Verification items for the finished model (mm, model axes). A direction names the side the tool comes from. Round coordinates to 2 decimals unless told otherwise and drop trailing zeros. Loops run counter-clockwise (first coordinate to the right, second up) from the corner with the lowest first, then second, coordinate; pieces in that order, holes last. Notation, with made-up numbers: M 12,-16.5 L 69,-16.5 A24 cw 69,5.5 Z; hole C -24.75,-6 d10. An arc over 180 degrees is marked long. Answer as CSV lines item,"result".
```python
from build123d import *

# Parameters (mm, degrees)
SKETCH1_W                = 6
SKETCH1_H                = 6
BOSS_EXTRUDE1_DEPTH      = 14
SKETCH2_W                = 1
SKETCH2_H                = 6
SKETCH2_W_2              = 1.5
BOSS_EXTRUDE2_DEPTH      = 10
FILLET1_R                = 3
SKETCH3_R                = 1.5
CUT_EXTRUDE1_DEPTH       = 10
CHAMFER1_SIZE            = 1
CHAMFER2_SIZE            = 1
FILLET1_OF_MIRROR2_R     = 3
CHAMFER1_OF_MIRROR2_SIZE = 1
SKETCH4_R                = 1.25
CUT_EXTRUDE2_DEPTH       = 13
CHAMFER3_SIZE            = 1
CUT_EXTRUDE3_DEPTH       = 10
CUT_EXTRUDE3_DEPTH_BACK  = 10
SKETCH5_W                = 10
SKETCH5_H                = 0.25
CUT_EXTRUDE4_DEPTH       = 10
CUT_EXTRUDE4_DEPTH_BACK  = 10
SKETCH6_W                = 10
SKETCH6_H                = 0.25
CHAMFER4_SIZE            = 1


with BuildPart() as part:
    # Sketch1 → Boss-Extrude1 (new body)
    with BuildSketch(Plane(origin=(0, 0, 0), x_dir=(0, 0, -1), z_dir=(1, 0, 0))):
        Rectangle(SKETCH1_W, SKETCH1_H)
    boss_extrude1 = extrude(amount=BOSS_EXTRUDE1_DEPTH)

    # Sketch2 → Boss-Extrude2 (add)
    with BuildSketch(Plane(origin=(14, 0, 0), x_dir=(0, 0, -1), z_dir=(1, 0, 0))):
        with Locations((3.5, 0)):
            Rectangle(SKETCH2_W, SKETCH2_H)
        with Locations((2.25, 0)):
            Rectangle(SKETCH2_W_2, SKETCH2_H)
    boss_extrude2 = extrude(amount=BOSS_EXTRUDE2_DEPTH)

    # Fillet1
    fillet1_edges = [part.edges().sort_by_distance(p)[0] for p in [
        (24, 3, -2.75),
        (24, -3, -2.75),
    ]]
    fillet(fillet1_edges, radius=FILLET1_R - 0.0001)  # a hair under: the kernel refuses the full size

    # Sketch3 → Cut-Extrude1 (cut)
    with BuildSketch(Plane(origin=(0, 0, -4), x_dir=(-1, 0, 0), z_dir=(0, 0, -1))):
        with Locations((-21, 0)):
            Circle(SKETCH3_R)
    cut_extrude1 = extrude(amount=-CUT_EXTRUDE1_DEPTH, mode=Mode.SUBTRACT)

    # Chamfer1
    chamfer1_edges = [part.edges().sort_by_distance(p)[0] for p in [
        (14, 0, -4),
    ]]
    chamfer(chamfer1_edges, length=CHAMFER1_SIZE - 0.0001)  # a hair under: the kernel refuses the full size

    # Chamfer2
    chamfer2_edges = [part.edges().sort_by_distance(p)[0] for p in [
        (14, 3, 0.75),
        (14, -3, 0.75),
    ]]
    chamfer(chamfer2_edges, length=CHAMFER2_SIZE)

    # Mirror2: Boss-Extrude1, Boss-Extrude2, Cut-Extrude1 across plane
    add(boss_extrude1.mirror(Plane(origin=(0, 0, 0), x_dir=(1, 0, 0), z_dir=(0, 0, -1))))
    add(boss_extrude2.mirror(Plane(origin=(0, 0, 0), x_dir=(1, 0, 0), z_dir=(0, 0, -1))))
    add(cut_extrude1.mirror(Plane(origin=(0, 0, 0), x_dir=(1, 0, 0), z_dir=(0, 0, -1))), mode=Mode.SUBTRACT)

    # Fillet1 of Mirror2
    fillet1_of_mirror2_edges = [part.edges().sort_by_distance(p)[0] for p in [
        (24, 3, 2.75),
        (24, -3, 2.75),
    ]]
    fillet(fillet1_of_mirror2_edges, radius=FILLET1_OF_MIRROR2_R - 0.0001)  # a hair under: the kernel refuses the full size

    # Chamfer1 of Mirror2
    chamfer1_of_mirror2_edges = [part.edges().sort_by_distance(p)[0] for p in [
        (14, 0, 4),
    ]]
    chamfer(chamfer1_of_mirror2_edges, length=CHAMFER1_OF_MIRROR2_SIZE - 0.0001)  # a hair under: the kernel refuses the full size

    # Sketch4 → Cut-Extrude2 (cut)
    with BuildSketch(Plane.ZY):
        Circle(SKETCH4_R)
    extrude(amount=-CUT_EXTRUDE2_DEPTH, mode=Mode.SUBTRACT)

    # Chamfer3
    chamfer3_edges = [part.edges().sort_by_distance(p)[0] for p in [
        (14, -3, 0),
        (14, 3, 0),
    ]]
    chamfer(chamfer3_edges, length=CHAMFER3_SIZE)

    # Sketch5 → Cut-Extrude3 (cut, two sides: drawn at the far end of the back side and taken through both)
    with BuildSketch(Plane(origin=(0, 0, 0), x_dir=(1, 0, 0), z_dir=(0, 1, 0)).offset(-CUT_EXTRUDE3_DEPTH_BACK)):
        with Locations((19, -1.625)):
            Rectangle(SKETCH5_W, SKETCH5_H)
    extrude(amount=CUT_EXTRUDE3_DEPTH + CUT_EXTRUDE3_DEPTH_BACK, mode=Mode.SUBTRACT)

    # Sketch6 → Cut-Extrude4 (cut, two sides: drawn at the far end of the back side and taken through both)
    with BuildSketch(Plane(origin=(0, 0, 0), x_dir=(1, 0, 0), z_dir=(0, 1, 0)).offset(-CUT_EXTRUDE4_DEPTH_BACK)):
        with Locations((19, 1.625)):
            Rectangle(SKETCH6_W, SKETCH6_H)
    extrude(amount=CUT_EXTRUDE4_DEPTH + CUT_EXTRUDE4_DEPTH_BACK, mode=Mode.SUBTRACT)

    # Chamfer4
    chamfer4_edges = [part.edges().sort_by_distance(p)[0] for p in [
        (14, -3, 1.625),
        (14, -3, -1.625),
        (14, 3, -1.625),
        (14, 3, 1.625),
    ]]
    chamfer(chamfer4_edges, length=CHAMFER4_SIZE - 0.0001)  # a hair under: the kernel refuses the full size


solid = part.part
```
1) Material ranges on probe 1 along X at (y, z) = (0, 2.2); probe 2 along Y at (x, z) = (6, 0); probe 3 along Z at (x, y) = (16.25, 2.75), recorded low to high.
Here are the results:
probe 1,"x = 0 to 19.5, 22.5 to 24"
probe 2,"y = -3 to -1.25, 1.25 to 3"
probe 3,"z = -4 to -1.75, 1.75 to 4"
2) Draft check along Z on faces 1 (the flat face through (18, 0, 4)), 2 (the flat face through (10, 3, 0)), 3 (the flat face through (13, 0, 0)). Enter one of: +Z half, -Z half, draft (parallel to the pull), parting line (faces both ways), or undercut.
Here are the results:
face 1,"+Z half"
face 2,"draft"
face 3,"undercut"
3) Go/stop test with flat-tipped pins: pin 1 (0.8 mm diameter, centred on x = 13.5, y = -2.5, fed in from +Z); pin 2 (3 mm diameter, centred on x = 9.5, y = -1, fed in from -Z); pin 3 (1.5 mm diameter, centred on y = -2.5, z = -2, fed in from -X); pin 4 (1.1 mm diameter, centred on x = 13.5, y = 2.5, fed in from +Z). Record where each tip stops, or that it passes through.
Here are the results:
pin 1,"stops at z = 3"
pin 2,"stops at z = -3"
pin 3,"stops at x = 0"
pin 4,"stops at z = 3.05"
4) Section check D-D (x = 20.75). Record the cut outline in (y, z), plus the area to 3 significant figures.
Here are the results:
outline,"M -3,-4 L -1.48,-4 L -1.48,-1.75 L -3,-1.75 Z; M -3,1.75 L -1.48,1.75 L -1.48,4 L -3,4 Z; M 1.48,-4 L 3,-4 L 3,-1.75 L 1.48,-1.75 Z; M 1.48,1.75 L 3,1.75 L 3,4 L 1.48,4 Z"
area,"13.7 mm^2"
5) Section check B-B (y = 1). State how many separate pieces and enclosed holes the cut face has, plus the area to 3 significant figures.
Here are the results:
separate pieces,"3"
enclosed holes,"0"
area,"97.7 mm^2"
6) Set-up check for faces 4 (the flat face through (14, 0, 0)), 5 (the cylindrical face through (6.41, -1.22, -0.27)), 6 (the cylindrical face through (23.14, 2.1, 2.86)): record each of +Z, -Z, +X, -X, +Y, -Y from which the full face is reachable in a straight line by a thin tool's end or side.
Here are the results:
face 4,"+X, +Y, -Y"
face 5,"-X"
face 6,"+Z, -Z, +X, +Y"
7) Section check A-A (x = 17.75). Record the cut outline in (y, z).
Here are the results:
outline,"M -3,-4 L 3,-4 L 3,-1.75 L -3,-1.75 Z; M -3,1.75 L 3,1.75 L 3,4 L -3,4 Z"
8) Section check C-C (z = 0). Record the cut outline in (x, y), plus the area to 3 significant figures.
Here are the results:
outline,"M 0,-3 L 13,-3 L 14,-2 L 14,2 L 13,3 L 0,3 L 0,1.25 L 13,1.25 L 13,-1.25 L 0,-1.25 Z"
area,"50.5 mm^2"
